CAD build for the part. Positions are in the model's coordinates, mm. Face numbers are marked on the shaded views. A direction names the side the tool comes from. Coordinates: 2 decimals unless noted, no trailing zeros. Order: outer loops, then holes, each group sorted by start corner. A loop starts at its lowest first (then second) coordinate and runs counter-clockwise, first axis right, second up. Notation, with made-up numbers: M 78,65 L 130,65 A20 cw 130,82 Z; hole C 34,43.25 d7. An arc over 180 degrees is marked long. Write item = value, one per line.
Autodesk Inventor part; units mm, degrees
ref_plane "YZ Plane" through (0, 0, 0) normal (1, 0, 0) x (0, 1, 0)
ref_plane "XZ Plane" through (0, 0, 0) normal (0, 1, 0) x (-1, 0, 0)
ref_plane "XY Plane" through (0, 0, 0) normal (0, 0, 1) x (1, 0, 0)
sketch "Sketch1" plane through (0, 0, 0) normal (0, 1, 0) x (-1, 0, 0)
  line L0 (3, -9.02) -> (33.75, -9.02)
  line L1 (33.75, -9.02) -> (33.75, 0)
  line L2 (33.75, 0) -> (36.75, 0)
  line L3 (36.75, 0) -> (36.75, -22.86)
  line L4 (36.75, -22.86) -> (22.375, -22.86)
  line L5 (22.375, -22.86) -> (22.375, -65.9087)
  line L6 (14.375, -22.86) -> (14.375, -65.9087)
  line L7 (18.375, -22.86) -> (18.375, -72.86) construction
  arc A0 (14.375, -65.9087) -> (22.375, -65.9087) centre (18.375, -72.86) ccw
  line L8 (3, -9.02) -> (3, 0)
  line L9 (3, 0) -> (0, 0)
  line L10 (0, 0) -> (0, -22.86)
  line L11 (14.375, -22.86) -> (0, -22.86)
  dimension "d2" = 30.75
  dimension "d3" = 3
  dimension "d4" = 22.86
  dimension "d9" = 8
  dimension "d12" = 4
  dimension "d13" = 8.02
  dimension "d15" = 14.375
  dimension "d16" = 3
  dimension "d17" = 22.86
extrude "Extrusion1" add sketch "Sketch1" along normal blind 10
sketch "Sketch2" plane through (0, 0, 0) normal (1, 0, 0) x (0, 0, -1)
  circle A0 centre (5, 5) radius 1.5
  line L0 (0, 0) -> (0, 10)
  line L1 (0, 10) -> (22.86, 10)
  dimension "d23" = 5
  dimension "d24" = 5
  dimension "d25" = 3
extrude "Extrusion2" cut sketch "Sketch2" against normal blind 3
sketch "Sketch3" plane through (-36.75, 0, -22.86) normal (-1, 0, 0) x (0, 0, 1)
  circle A0 centre (17.86, 5) radius 1.5
  circle A1 centre (17.86, 5) radius 1.5
  point P0 (22.86, 0)
extrude "Extrusion3" cut sketch "Sketch3" against normal blind 3
sketch "Sketch4" plane through (0, 10, 0) normal (0, 1, 0) x (1, 0, 0)
  arc A0 (-14.375, 65.9087) -> (-22.375, 65.9087) centre (-18.375, 72.86) ccw
  circle A1 centre (-18.375, 72.86) radius 6.015
  point P0 (0, 0)
  dimension "d30" = 12.03
extrude "Extrusion4" cut sketch "Sketch4" against normal blind 5
fillet "Fillet1" radius 2 7 edges at (-18.375, 0, -80.88) (-14.375, 0, -44.3844) (-7.1875, 0, -22.86) (-29.5625, 0, -22.86) (0, 0, -11.43) (-36.75, 0, -11.43) (-22.375, 0, -44.3844)
properties part number "Tarea 16 P2"
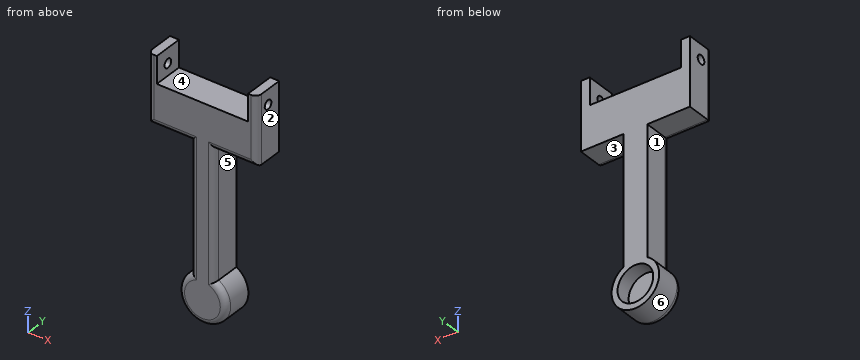
(1) Pin check, flat tips, straight feed: pin 1 Ø19 at (x, z) = (-18.375, -72.86) entering from -Y; pin 2 Ø2.5 at (y, z) = (7.5, -47.5) entering from +X (3 decimals); pin 3 Ø2.5 at (x, y) = (-10, 5.5) entering from -Z; pin 4 Ø2 at (x, y) = (-6.5, 8) entering from -Z. Stop position of each tip, or through.
Evaluation:
pin_1 = 0
pin_2 = -14.375
pin_3 = -76.54
pin_4 = -22.86
(2) Pull direction X, two halves, no side cores. Call the marked faces 3, 4, 5 and 6: +X half, -X half, draft (parallel to the pull), parting line (faces both ways), or undercut.
Evaluation:
face_3 = draft
face_4 = undercut
face_5 = +X half
face_6 = parting line
(3) Slice it at D-D, the plane z = -72.86. Write the cut outline in (x, y), then the cut area to 3 significant figures.
Evaluation:
outline = M -26.4,2 A2 ccw -24.4,0 L -12.35,0 A2 ccw -10.35,2 L -10.35,10 L -12.36,10 L -12.36,5 L -24.39,5 L -24.39,10 L -26.4,10 Z
area = 98.5 mm²
(4) Tool access for the marked faces 1 and 2: list every direction of +Z, -Z, +X, -X, +Y, -Y with a clear straight run to the whole face (end or side of a thin tool).
Evaluation:
face_1 = -X, +Y, -Y
face_2 = +Z, -Z, +X, +Y, -Y
(5) Slice it at B-B, the plane y = 9. Write the cut outline in (x, z) (3 decimals).
Evaluation:
outline = M -36.75,-22.86 L -22.375,-22.86 L -22.375,-65.909 A8.02 ccw long -14.375,-65.909 L -14.375,-22.86 L 0,-22.86 L 0,0 L -3,0 L -3,-9.02 L -33.75,-9.02 L -33.75,0 L -36.75,0 Z; hole C -18.375,-72.86 d12.03
(6) Slice it at A-A, the plane z = -5. Write the cut outline in (x, y), then the cut area to 3 significant figures.
Evaluation:
outline = M -36.75,2 A2 ccw -34.75,0 L -33.75,0 L -33.75,3.5 L -36.75,3.5 Z; M -36.75,6.5 L -33.75,6.5 L -33.75,10 L -36.75,10 Z; M -3,0 L -2,0 A2 ccw 0,2 L 0,3.5 L -3,3.5 Z; M -3,6.5 L 0,6.5 L 0,10 L -3,10 Z
area = 40.3 mm²
(7) Slice it at C-C, the plane z = -31.5. Write the cut outline in (x, y) (3 decimals).
Evaluation:
outline = M -22.375,2 A2 ccw -20.375,0 L -16.375,0 A2 ccw -14.375,2 L -14.375,10 L -22.375,10 Z
(8) Wall check: line 1 (Y direction, x = -35, z = -5); line 2 (X direction, y = 6.25, z = -8.5); line 3 (X direction, y = 8.9, z = -72.86). Give the ranges that are in metal, low to high. Write a range as from..to.
Evaluation:
line_1 = 0.02..3.5, 6.5..10
line_2 = -36.75..-33.75, -3..0
line_3 = -26.4..-24.39, -12.36..-10.35
